Can you work these out from the model? Positions are in its coordinate system, mm. Face numbers are marked on the shaded views. A direction names the side the tool comes from. Round coordinates to 2 decimals unless told otherwise and drop trailing zeros. Loops run counter-clockwise (first coordinate to the right, second up) from the corner with the lowest first, then second, coordinate; pieces in that order, holes last. Notation, with made-up numbers: (85, 56) -> (100, 56) arc R19 cw to (100, 64) -> close; hole circle Ø11 at (72.5, -11.75). An arc over 180 degrees is marked (long way). Use a Markdown table: item, result.
from build123d import *

# Parameters (mm, degrees)
RESSALTO_EXTRUS_O1_DEPTH = 6


with BuildPart() as part:
    # Model → Ressalto-extrusão1 (new body)
    with BuildSketch(Plane.XY):
        Polygon((36.978091014, 23.513650985), (35.70530016, 22.240860131), (39.311542875, 18.634617416), (40.584333729, 19.90740827), (43.377405166, 17.114336834), (46.488678057, 20.225609725), (43.695606621, 23.018681162), (44.968397475, 24.291472016), (41.36215476, 27.897714731), (40.089363906, 26.624923877), (36.341699099, 30.372588684), (40.614784991, 34.645674576), (36.134425304, 39.126034262), (49.852292818, 52.843901776), (54.332652505, 48.36354209), (73.636667559, 67.667557144), (73.636667559, 8.867561848), (60.3697662, 8.867561848), (60.3697662, 14.167560246), (62.169764288, 14.167560246), (62.169764288, 19.267557602), (60.3697662, 19.267557602), (60.3697662, 23.217557109), (55.96976188, 23.217557109), (55.96976188, 19.267557602), (54.169763792, 19.267557602), (54.169763792, 14.167560246), (55.96976188, 14.167560246), (55.96976188, 8.867561848), (32.16976612, 8.867561848), (32.16976612, 26.200655705), (33.230426207, 27.261315792), align=None)
        Polygon((60.386985649, 34.892299852), (66.57416949, 28.705116012), (61.712810758, 23.84375728), (56.542974359, 29.013593679), (56.37928278, 30.884596983), align=None, mode=Mode.SUBTRACT)
        Polygon((46.676618489, 24.010359591), (66.475606779, 43.80934788), (62.956288895, 47.328665763), (43.157300606, 27.529677474), align=None, mode=Mode.SUBTRACT)
    extrude(amount=RESSALTO_EXTRUS_O1_DEPTH)


solid = part.part
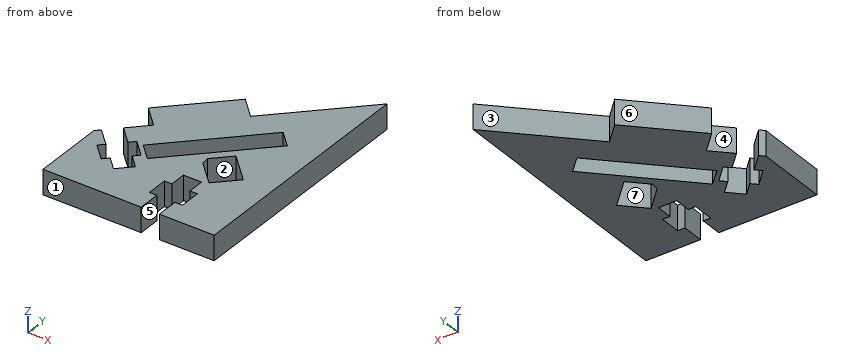
1. Will these pins go through, and if not, where does the flat tip stop? pin 1 Ø3 at (y, z) = (33.5, 3.5) entering from -X; pin 2 Ø4 at (x, y) = (41, 48) entering from +Z; pin 3 Ø2 at (x, z) = (61, 2) entering from +Y; pin 4 Ø10 at (x, y) = (40, 38) entering from -Z.
Answer sheet:
| item | result |
|---|---|
| pin 1 | stops at x = 37.97 |
| pin 2 | passes through |
| pin 3 | stops at y = 56.03 |
| pin 4 | stops at z = 0 |
2. I want a section at D-D (y = 45). Please give me the cut outline in (x, z), plus the area to 3 significant figures.
Answer sheet:
| item | result |
|---|---|
| outline | (42.01, 0) -> (60.63, 0) -> (60.63, 6) -> (42.01, 6) -> close; (65.28, 0) -> (73.64, 0) -> (73.64, 6) -> (65.28, 6) -> close |
| area | 162 mm² |
3. Which directions (+Z, -Z, +X, -X, +Y, -Y) give clear straight access to the entire face, cutting with the end or side of a thin tool? Please do the marked faces 1, 2, 3 and 4.
Answer sheet:
| item | result |
|---|---|
| face 1 | +Z, -Z, +X, -X, -Y |
| face 2 | +Z, -Z |
| face 3 | +Z, -Z, +Y |
| face 4 | +Z, -Z, -X |
4. I want a section at B-B (x = 53.5). Please give me the cut outline in (y, z), plus the area to 3 significant figures.
Answer sheet:
| item | result |
|---|---|
| outline | (8.87, 0) -> (30.83, 0) -> (30.83, 6) -> (8.87, 6) -> close; (37.87, 0) -> (49.2, 0) -> (49.2, 6) -> (37.87, 6) -> close |
| area | 200 mm² |
5. I need wall thicknesses on line 1 (Y direction, x = 60.5, z = 2.45); line 2 (X direction, y = 27.5, z = 2.15); line 3 (X direction, y = 17, z = 0.5). Which ranges of each line are inside material? Lowest first, please.
Answer sheet:
| item | result |
|---|---|
| line 1 | y = 8.87 to 14.17, 19.27 to 25.06, 34.78 to 37.83, 44.87 to 54.53 |
| line 2 | x = 39.21 to 40.96, 41.76 to 43.19, 50.17 to 58.06, 65.37 to 73.64 |
| line 3 | x = 32.17 to 54.17, 62.17 to 73.64 |
6. I want a section at A-A (y = 33). Please give me the cut outline in (x, z).
Answer sheet:
| item | result |
|---|---|
| outline | (38.97, 0) -> (48.63, 0) -> (48.63, 6) -> (38.97, 6) -> close; (55.67, 0) -> (58.49, 0) -> (58.49, 6) -> (55.67, 6) -> close; (62.28, 0) -> (73.64, 0) -> (73.64, 6) -> (62.28, 6) -> close |
7. If we mould it in two halves opening along Y, with no side actions, what happens to the marked faces 5, 6 and 7? For each: +Y half, -Y half, draft (parallel to the pull), parting line (faces both ways), or undercut.
Answer sheet:
| item | result |
|---|---|
| face 5 | draft |
| face 6 | +Y half |
| face 7 | undercut |
8. I want a section at C-C (x = 65.5). Please give me the cut outline in (y, z).
Answer sheet:
| item | result |
|---|---|
| outline | (8.87, 0) -> (27.63, 0) -> (27.63, 6) -> (8.87, 6) -> close; (29.78, 0) -> (42.83, 0) -> (42.83, 6) -> (29.78, 6) -> close; (44.78, 0) -> (59.53, 0) -> (59.53, 6) -> (44.78, 6) -> close |
